from build123d import *

# Parameters (mm, degrees)
SKETCH1_R           = 2
BOSS_EXTRUDE1_DEPTH = 3
SKETCH2_R           = 1.1303
CUT_EXTRUDE1_DEPTH  = 41.422765863
BOSS_EXTRUDE4_DEPTH = 3
FILLET1_R           = 5


with BuildPart() as part:
    # Sketch1 → Boss-Extrude1 (new body)
    with BuildSketch(Plane(origin=(0, 0, 0), x_dir=(0, 0, -1), z_dir=(1, 0, 0))):
        Polygon((-5, 5), (35, 5), (35, -5), (5, -5), (5, -20), (-5, -20), align=None)
        Circle(SKETCH1_R, mode=Mode.SUBTRACT)
    extrude(amount=BOSS_EXTRUDE1_DEPTH)

    # Sketch2 → Cut-Extrude1 (cut, through all)
    with BuildSketch(Plane(origin=(3, 0, 0), x_dir=(0, 0, -1), z_dir=(1, 0, 0))):
        with Locations((-1.7, -15.5)):
            Circle(SKETCH2_R)
    extrude(amount=-CUT_EXTRUDE1_DEPTH, mode=Mode.SUBTRACT)

    # Sketch3 → Boss-Extrude4 (add)
    with BuildSketch(Plane(origin=(3, 0, 0), x_dir=(0, 0, -1), z_dir=(1, 0, 0))):
        with BuildLine():
            Line((-5, -18), (-5, -13))
            add(Edge.make_bspline(
                [(-5, -13), (-5.721407716, -15.082195162), (-10.455731115, -13.770011947), (-10.499261295, -15.5)],
                knots=[0, 0, 0, 0, 1, 1, 1, 1], degree=3))
            add(Edge.make_bspline(
                [(-5, -18), (-5.721407716, -15.917804838), (-10.455731115, -17.229988053), (-10.499261295, -15.5)],
                knots=[0, 0, 0, 0, 1, 1, 1, 1], degree=3))
        make_face()
    extrude(amount=-BOSS_EXTRUDE4_DEPTH)

    # Fillet1
    # the kernel refuses this fillet: 5 mm, written as the material it adds along each edge
    with BuildSketch(Plane(origin=(0, -5, -5), x_dir=(0, 0, -1), z_dir=(1, 0, 0))) as fillet1_piece_1:
        with BuildLine():
            CenterArc((FILLET1_R, -FILLET1_R), FILLET1_R, 90, 90)
            Line((0, -FILLET1_R), (0, 0))
            Line((0, 0), (FILLET1_R, 0))
        make_face()
    extrude(amount=3)
    # the kernel refuses this fillet: 5 mm, written as the material it takes off along each edge
    with BuildSketch(Plane(origin=(-12.5, -20, -5), x_dir=(0, 1, 0), z_dir=(1, 0, 0)), Plane(origin=(-12.5, -5, -35), x_dir=(0, 1, 0), z_dir=(1, 0, 0)), Plane(origin=(-12.5, 5, -35), x_dir=(0, 0, 1), z_dir=(1, 0, 0))) as fillet1_2_piece_1:
        with BuildLine():
            CenterArc((FILLET1_R, FILLET1_R), FILLET1_R, 180, 90)
            Line((0, FILLET1_R), (0, 0))
            Line((0, 0), (FILLET1_R, 0))
        make_face()
    extrude(amount=28, mode=Mode.SUBTRACT)
    with BuildSketch(Plane(origin=(-12.5, 5, 5), x_dir=(0, 0, -1), z_dir=(1, 0, 0))) as fillet1_2_piece_2:
        with BuildLine():
            CenterArc((FILLET1_R, -FILLET1_R), FILLET1_R, 90, 90)
            Line((0, -FILLET1_R), (0, 0))
            Line((0, 0), (FILLET1_R, 0))
        make_face()
    extrude(amount=28, mode=Mode.SUBTRACT)
    with BuildSketch(Plane(origin=(-10, -20, 5), x_dir=(0, 0, -1), z_dir=(1, 0, 0))) as fillet1_2_piece_3:
        with BuildLine():
            CenterArc((4, 5), FILLET1_R, 216.869897646, 53.130102354)
            Line((0, 2), (0, 0))
            Line((0, 0), (4, 0))
        make_face()
    extrude(amount=23, mode=Mode.SUBTRACT)


solid = part.part
Input: part model. Units: mm. Frame: model coordinates. A direction names the side the tool comes from. Coordinates: 2 decimals unless noted, no trailing zeros. Loops run counter-clockwise (first coordinate to the right, second up) from the corner with the lowest first, then second, coordinate; pieces in that order, holes last.
(1) Material intervals for probe 1 along Y at (x, z) = (2.35, 0); probe 2 along Z at (x, y) = (2.3, -16.25); probe 3 along Z at (x, y) = (2.55, -15), sorted ascending.
(2) Pull-direction query (Y, two-part tool) for faces 1 (the face through (1, -19, -3)), 2 (the face through (1, -2, 0)), 3 (the face through (1, 0, -35)); classes: released by +Y, released by -Y, zero draft, split by the parting line, or undercut.
(3) Section B-B on z = -17.5. Return the cut outline in (x, y).
(4) Section A-A on x = 1.6. Count the separate pieces of the cut face and the enclosed holes in it, then the cut area to 3 significant figures.
(5) Section C-C on y = -4. Return the cut outline in (x, z), then the cut area to 3 significant figures.
(6) Set-up query: faces 4 (the face through (1, -7, 5)), 5 (the face through (1, -12, -5)), 6 (the face through (3, -4.5, -12.6)). Return all of +Z, -Z, +X, -X, +Y, -Y with unobstructed straight access to the full face (end or side cutting, diameter ignored); none if empty.
Data:
1. probe 1: y = -20 to -2, 2 to 5
1. probe 2: z = -4.84 to 0.85, 2.55 to 9.93
1. probe 3: z = -5 to 0.69, 2.71 to 10.3
2. face 1: released by -Y
2. face 2: undercut
2. face 3: split by the parting line
3. outline: (0, -5) - (3, -5) - (3, 5) - (0, 5) - close
4. separate pieces: 1
4. enclosed holes: 2
4. area: 528 mm2
5. outline: (0, -33) - (3, -33) - (3, 5) - (0, 5) - close
5. area: 114 mm2
6. face 4: +Z, +X, -X, +Y
6. face 5: -Z, +X, -X, -Y
6. face 6: +Z, -Z, +X, +Y, -Y
